```python
from build123d import *

# Parameters (mm, degrees)
SKETCH_1_W             = 207
SKETCH_1_H             = 210
EXTRUDE_1_DEPTH        = 6
SKETCH_2_R             = 3.3
CUT_EXTRUDE_1_DEPTH    = 148.557615866
CHAMFER_2_SIZE         = 5
CHAMFER_1_SIZE         = 1
HOLE_WIZARD_M4_1_D     = 3.3
HOLE_WIZARD_M4_1_DEPTH = 10.1
HOLE_WIZARD_M4_1_TIP   = 0.991420021
HOLE_WIZARD_M3_1_D     = 2.5
HOLE_WIZARD_M3_1_DEPTH = 7.5
HOLE_WIZARD_M3_1_TIP   = 0.751075774
SKETCH_7_R             = 12.5
CUT_EXTRUDE_2_DEPTH    = 148.557615866
SKETCH_8_R             = 12.5
CUT_EXTRUDE_3_DEPTH    = 148.557615866
CUT_EXTRUDE_4_DEPTH    = 148.557615866
CHAMFER_3_SIZE         = 1


with BuildPart() as part:
    # 草图1 → 凸台-拉伸1 (new body)
    with BuildSketch(Plane.XY):
        Rectangle(SKETCH_1_W, SKETCH_1_H)
    extrude(amount=EXTRUDE_1_DEPTH)

    # 草图2 → 切除-拉伸1 (cut, through all)
    with BuildSketch(Plane.XY.offset(6)):
        with Locations((-78.5, 97)):
            Circle(SKETCH_2_R)
        with Locations((78.5, 97)):
            Circle(SKETCH_2_R)
        with Locations((-78.5, -97)):
            Circle(SKETCH_2_R)
        with Locations((78.5, -97)):
            Circle(SKETCH_2_R)
    extrude(amount=-CUT_EXTRUDE_1_DEPTH, mode=Mode.SUBTRACT)

    # 倒角2
    chamfer_2_edges = [part.edges().sort_by_distance(p)[0] for p in [
        (103.5, -105, 3),
        (-103.5, -105, 3),
        (-103.5, 105, 3),
        (103.5, 105, 3),
    ]]
    chamfer(chamfer_2_edges, length=CHAMFER_2_SIZE)

    # 倒角1
    chamfer_1_edges = [part.edges().sort_by_distance(p)[0] for p in [
        (0, -105, 0),
        (0, -105, 6),
        (103.5, 0, 0),
        (-103.5, 0, 0),
        (0, 105, 0),
        (101, 102.5, 0),
        (-101, 102.5, 0),
        (101, -102.5, 0),
        (-101, -102.5, 0),
        (-103.5, 0, 6),
        (103.5, 0, 6),
        (0, 105, 6),
        (101, 102.5, 6),
        (-101, 102.5, 6),
        (101, -102.5, 6),
        (-101, -102.5, 6),
    ]]
    chamfer(chamfer_1_edges, length=CHAMFER_1_SIZE)

    # M4 螺纹孔1
    with Locations(Plane(origin=(0, 0, 0), x_dir=(-1, 0, 0), z_dir=(0, 0, -1))):
        with Locations((-16, 14), (16, 14), (16, -69), (-16, -69)):
            Hole(HOLE_WIZARD_M4_1_D / 2, depth=HOLE_WIZARD_M4_1_DEPTH)
            with Locations((0, 0, -(HOLE_WIZARD_M4_1_DEPTH + HOLE_WIZARD_M4_1_TIP / 2))):  # 118° drill point
                Cone(0, HOLE_WIZARD_M4_1_D / 2, HOLE_WIZARD_M4_1_TIP, mode=Mode.SUBTRACT)

    # M3 螺纹孔1
    with Locations(Plane(origin=(0, 0, 0), x_dir=(-1, 0, 0), z_dir=(0, 0, -1))):
        with Locations((0, 58), (0, 88)):
            Hole(HOLE_WIZARD_M3_1_D / 2, depth=HOLE_WIZARD_M3_1_DEPTH)
            with Locations((0, 0, -(HOLE_WIZARD_M3_1_DEPTH + HOLE_WIZARD_M3_1_TIP / 2))):  # 118° drill point
                Cone(0, HOLE_WIZARD_M3_1_D / 2, HOLE_WIZARD_M3_1_TIP, mode=Mode.SUBTRACT)

    # 草图7 → 切除-拉伸2 (cut, through all)
    with BuildSketch(Plane(origin=(0, 0, 0), x_dir=(-1, 0, 0), z_dir=(0, 0, -1))):
        with Locations((0, 73)):
            Circle(SKETCH_7_R)
    extrude(amount=-CUT_EXTRUDE_2_DEPTH, mode=Mode.SUBTRACT)

    # 草图8 → 切除-拉伸3 (cut, through all)
    with BuildSketch(Plane(origin=(0, 0, 0), x_dir=(-1, 0, 0), z_dir=(0, 0, -1))):
        with Locations((0, -27.5)):
            Circle(SKETCH_8_R)
    extrude(amount=-CUT_EXTRUDE_3_DEPTH, mode=Mode.SUBTRACT)

    # 草图9 → 切除-拉伸4 (cut, through all)
    with BuildSketch(Plane(origin=(0, 0, 0), x_dir=(-1, 0, 0), z_dir=(0, 0, -1))):
        with BuildLine():
            Line((-87.5, -65), (-87.5, 65))
            ThreePointArc((-87.5, 65), (-70, 82.5), (-52.5, 65))
            Line((-52.5, 65), (-52.5, -65))
            ThreePointArc((-52.5, -65), (-70, -82.5), (-87.5, -65))
        make_face()
        with BuildLine():
            Line((52.5, -65), (52.5, 65))
            ThreePointArc((52.5, 65), (70, 82.5), (87.5, 65))
            Line((87.5, 65), (87.5, -65))
            ThreePointArc((87.5, -65), (70, -82.5), (52.5, -65))
        make_face()
    extrude(amount=-CUT_EXTRUDE_4_DEPTH, mode=Mode.SUBTRACT)

    # 倒角3
    chamfer_3_edges = [part.edges().sort_by_distance(p)[0] for p in [
        (12.5, 73, 6),
        (12.5, 73, 0),
        (12.5, -27.5, 6),
        (12.5, -27.5, 0),
        (70, -82.5, 6),
        (87.5, 0, 6),
        (70, 82.5, 6),
        (52.5, 0, 6),
        (70, -82.5, 0),
        (52.5, 0, 0),
        (70, 82.5, 0),
        (87.5, 0, 0),
        (-70, -82.5, 6),
        (-52.5, 0, 6),
        (-70, 82.5, 6),
        (-87.5, 0, 6),
        (-70, -82.5, 0),
        (-87.5, 0, 0),
        (-70, 82.5, 0),
        (-52.5, 0, 0),
    ]]
    chamfer(chamfer_3_edges, length=CHAMFER_3_SIZE)


solid = part.part
```
Could you check a few things on this model? Use its own coordinates, in mm. A direction names the side the tool comes from. Coordinates: 2 decimals unless noted, no trailing zeros. Loops run counter-clockwise (first coordinate to the right, second up) from the corner with the lowest first, then second, coordinate; pieces in that order, holes last. Notation, with made-up numbers: M -30.75,-9.75 L 12.25,-9.75 A20 ccw 12.25,26.25 Z; hole C 86,25 d9. An arc over 180 degrees is marked long. Put each result on its own line as item: value. Start each with the question number.
(1) Suppose I cut it at A-A on y = -27.5. Count the separate pieces of the cut face and the enclosed holes in it, then the cut area to 3 significant figures.
(2) Thinking about a two-plate mould opening in Y: for faces 5 (the face through (70.388, -82.655, 5.16)), 6 (the face through (69.615, -82.496, 2.972)), 7 (the face through (100.62, -102.19, 5.49)), 8 (the face through (100.62, 102.19, 0.51)), which applies, pulls with the +Y half, pulls with the -Y half, needs draft (parallel to the pull), parting line crosses it, or undercut?
(3) Suppose I cut it at C-C on y = 20.5. Please give me the cut outline in (x, z), then the cut area to 3 significant figures.
(4) I need wall thicknesses on line 1 (X direction, y = 33, z = 2.5); line 2 (Y direction, x = 16, z = 3.25); line 3 (Y direction, x = 78.5, z = 3.9). Which ranges of each line are inside material? Lowest first, please. Write a range as from..to.
(5) For faces 1 (the face through (69.612, 82.655, 5.16)), 2 (the face through (100.62, -102.19, 0.51)), 3 (the face through (-69.615, 82.496, 2.972)), 4 (the face through (-69.612, 82.655, 0.84)), which set-ups out of +Z, -Z, +X, -X, +Y, -Y let a thin tool reach every point of the face, with its end or its side?
(6) Will this pin go through, and if not, where does the flat tip stop? P1, Ø20, axis at x = 0, y = 73, coming from the +Z side.
Solutions:
1. separate pieces: 4
1. enclosed holes: 0
1. area: 664 mm2
2. face 5: undercut
2. face 6: undercut
2. face 7: pulls with the -Y half
2. face 8: pulls with the +Y half
3. outline: M -103.5,1 L -102.5,0 L -88.5,0 L -87.5,1 L -87.5,5 L -88.5,6 L -102.5,6 L -103.5,5 Z; M -52.5,1 L -51.5,0 L 51.5,0 L 52.5,1 L 52.5,5 L 51.5,6 L -51.5,6 L -52.5,5 Z; M 87.5,1 L 88.5,0 L 102.5,0 L 103.5,1 L 103.5,5 L 102.5,6 L 88.5,6 L 87.5,5 Z
3. area: 816 mm2
4. line 1: x = -103.5..-87.5, -52.5..52.5, 87.5..103.5
4. line 2: y = -105..-70.65, -67.35..12.35, 15.65..105
4. line 3: y = -105..-100.3, -93.7..-80.3, 80.3..93.7, 100.3..105
5. face 1: +Z
5. face 2: -Z, +X, -Y
5. face 3: +Z, -Z
5. face 4: -Z
6. P1: passes through
